Geometry check sheet. Reference: the model listing, model coordinates, mm. A direction names the side the tool comes from. Round coordinates to 2 decimals unless told otherwise and drop trailing zeros. Write each loop counter-clockwise with the first axis right and the second up, starting at its lowest first coordinate (ties: lowest second). Pieces come first, ordered by that corner, then holes. Notation, with made-up numbers: (69.25, -5.5) - (119.25, -5.5) arc R18 ccw to (119.25, 0.5) - close; hole circle Ø4 at (-29.75, 89). An arc over 180 degrees is marked (long way). One line per question, with ' | ' between items. Start each with the question number.
from build123d import *

# Parameters (mm, degrees)
F1_DEPTH = 25


with BuildPart() as f1:
    # F0 (on Front) → F1 (new body)
    with BuildSketch(Plane.XZ):
        Polygon((225, 186), (0, 186), (-225, 186), (-225, 180), (-250, 180), (-250, 125.809848), (-225, 100.809848), (-250, 75.809848), (-250, 0), (-250, -75.809848), (-225, -100.809848), (-250, -125.809848), (-250, -180), (-225, -180), (-225, -186), (0, -186), (225, -186), (225, -180), (250, -180), (250, -125.809848), (225, -100.809848), (250, -75.809848), (250, 0), (250, 75.809848), (225, 100.809848), (250, 125.809848), (250, 180), (225, 180), align=None)
    extrude(amount=F1_DEPTH)


solid = f1.part
Q1. Go/stop test with flat-tipped pins: P1, Ø12.5, axis at x = -232.5, y = -11, coming from the -Z side; P2, Ø3, axis at y = -16, z = 184, coming from the +X side; P3, Ø12.5, axis at x = -241, y = -14.5, coming from the +Z side. Record where each tip stops, or that it passes through.
Q2. Section check A-A, the plane y = -14.5. Record the cut outline in (x, z).
Q3. Draft check along Z on faces 1 (the flat face through (237.325, -12.325, -88.485)), 2 (the flat face through (237.675, -12.325, -113.485)), 3 (the flat face through (-237, -12, 180)), 4 (the flat face through (237, -12, -180)). Enter one of: pulls with the +Z half, pulls with the -Z half, needs draft (parallel to the pull), parting line crosses it, or undercut.
Q4. Thickness scan on line 1 (X direction, y = -2.75, z = -121). Record the ranges inside material, lowest first.
Q5. Set-up check for faces 5 (the flat face through (238, -12, 180)), 6 (the flat face through (-237.675, -12.325, 113.485)), 7 (the flat face through (237.32, -12.32, 113.13)): record each of +Z, -Z, +X, -X, +Y, -Y from which the full face is reachable in a straight line by a thin tool's end or side.
Result sheet:
1) P1: z = -180 | P2: x = 225 | P3: z = 180
2) outline: (-250, -180) - (-225, -180) - (-225, -186) - (225, -186) - (225, -180) - (250, -180) - (250, -125.81) - (225, -100.81) - (250, -75.81) - (250, 75.81) - (225, 100.81) - (250, 125.81) - (250, 180) - (225, 180) - (225, 186) - (-225, 186) - (-225, 180) - (-250, 180) - (-250, 125.81) - (-225, 100.81) - (-250, 75.81) - (-250, -75.81) - (-225, -100.81) - (-250, -125.81) - close
3) face 1: undercut | face 2: undercut | face 3: pulls with the +Z half | face 4: pulls with the -Z half
4) line 1: -245.19 to 245.19
5) face 5: +Z, +X, +Y, -Y | face 6: -X, +Y, -Y | face 7: +X, +Y, -Y
